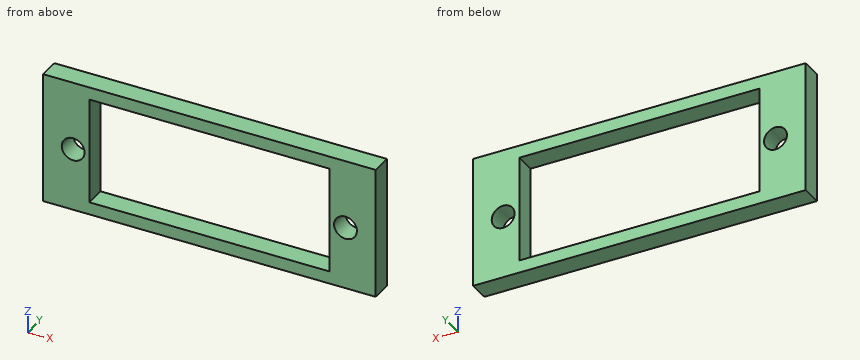
```python
from build123d import *

# Parameters (mm, degrees)
SCHIZZO1_W                   = 32
SCHIZZO1_H                   = 12.6
SCHIZZO1_R                   = 1.1
SCHIZZO1_W_2                 = 23.1
SCHIZZO1_H_2                 = 10.2
ESTRUSIONE_ESTRUSIONE1_DEPTH = 2


with BuildPart() as part:
    # Schizzo1 → Estrusione-Estrusione1 (new body)
    with BuildSketch(Plane(origin=(0, 0, 0), x_dir=(1, 0, 0), z_dir=(0, 1, 0))):
        with Locations((16, 6.3)):
            Rectangle(SCHIZZO1_W, SCHIZZO1_H)
        with Locations(Location((2.9, 6.6, 0), (0, 0, 270))):
            Circle(SCHIZZO1_R, mode=Mode.SUBTRACT)
        with Locations(Location((29.1, 6.6, 0), (0, 0, 270))):
            Circle(SCHIZZO1_R, mode=Mode.SUBTRACT)
        with Locations((16, 6.3)):
            Rectangle(SCHIZZO1_W_2, SCHIZZO1_H_2, mode=Mode.SUBTRACT)
    extrude(amount=ESTRUSIONE_ESTRUSIONE1_DEPTH)


solid = part.part
```
Build history of the part. All positions in model axes, mm. Give positions to 0.01 mm unless a question says otherwise; leave off trailing zeros. Loops run counter-clockwise (first coordinate to the right, second up) from the corner with the lowest first, then second, coordinate; pieces in that order, holes last.
1) Band-saw the part on C-C on z = -6.6. List the corners of the cut face in (x, y).
Values follow:
outline: (0, 0) - (1.8, 0) - (1.8, 2) - (0, 2) - close; (4, 0) - (4.45, 0) - (4.45, 2) - (4, 2) - close; (27.55, 0) - (28, 0) - (28, 2) - (27.55, 2) - close; (30.2, 0) - (32, 0) - (32, 2) - (30.2, 2) - close
2) Probe line 1 along X through (y, z) = (0.4, -6.6); line 2 along Z through (x, y) = (24, 1.7); line 3 along X through (y, z) = (1.3, -9). List the from-to ranges inside material, lowest first.
Values follow:
line 1: x = 0 to 1.8, 4 to 4.45, 27.55 to 28, 30.2 to 32
line 2: z = -12.6 to -11.4, -1.2 to 0
line 3: x = 0 to 4.45, 27.55 to 32
3) Band-saw the part on A-A on x = 6. List the corners of the cut face in (y, z).
Values follow:
outline: (0, -12.6) - (2, -12.6) - (2, -11.4) - (0, -11.4) - close; (0, -1.2) - (2, -1.2) - (2, 0) - (0, 0) - close
4) Band-saw the part on B-B on z = -4. List the corners of the cut face in (x, y).
Values follow:
outline: (0, 0) - (4.45, 0) - (4.45, 2) - (0, 2) - close; (27.55, 0) - (32, 0) - (32, 2) - (27.55, 2) - close
5) Drop a flat-ended pin along its axis: P1, Ø2, axis at x = 29.1, z = -6.6, coming from the +Y side. Give the stop position or say it passes through.
Values follow:
P1: passes through
6) Band-saw the part on D-D on y = 0.95. List the corners of the cut face in (x, z), then the cut area to 3 significant figures.
Values follow:
outline: (0, -12.6) - (32, -12.6) - (32, 0) - (0, 0) - close; hole circle Ø2.2 at (2.9, -6.6); hole (4.45, -11.4) - (27.55, -11.4) - (27.55, -1.2) - (4.45, -1.2) - close; hole circle Ø2.2 at (29.1, -6.6)
area: 160 mm2
